Check sheet for the drawn part. Datum: minimum x, y, z corner. Units: mm. A direction names the side the tool comes from. Coordinates: 2 decimals unless noted, no trailing zeros. Write each loop counter-clockwise with the first axis right and the second up, starting at its lowest first coordinate (ties: lowest second). Pieces come first, ordered by that corner, then holes. Notation, with made-up numbers: (14, -18.75) - (57, -18.75) arc R13 cw to (57, 5.25) - close; hole circle Ø2 at (54, -4). An arc over 180 degrees is marked (long way). Use one line per item in the form item = value. Start each with the question number.
1. Cross-section at A-A on y = 4. Record the boundary of the cut face in (x, z).
2. Cross-section at C-C on z = 10.5. Record the boundary of the cut face in (x, y).
3. Scan lines: line 1 along Z through (x, y) = (56, 7.5); line 2 along Z through (x, y) = (39, 34); line 3 along X through (y, z) = (19.5, 13). Record each from-to range of solid material in increasing order.
4. Cross-section at B-B on y = 37.5. Record the boundary of the cut face in (x, z), then the cut area to 3 significant figures.
5. Tool access check on the marked faces 1, 2 and 3. Record the directions out of +Z, -Z, +X, -X, +Y, -Y that give a thin tool (end or side, any length) a straight path to the whole face; none if there is none.
6. Go/stop test with flat-tipped pins: pin 1 Ø1 at (x, z) = (43, 7.5) entering from +Y; pin 2 Ø5 at (x, y) = (8, 29.5) entering from +Z; pin 3 Ø3 at (x, z) = (63, 25.5) entering from +Y; pin 4 Ø1.5 at (y, z) = (14.5, 37.5) entering from +X. Record where each tip stops, or that it passes through.
7. Draft check along X on the marked faces 4, 5, 6 and 7. Enter one of: +X half, -X half, draft (parallel to the pull), parting line (faces both ways), or undercut.
8. Cross-section at D-D on z = 24. Record the boundary of the cut face in (x, y), then the cut area to 3 significant figures.
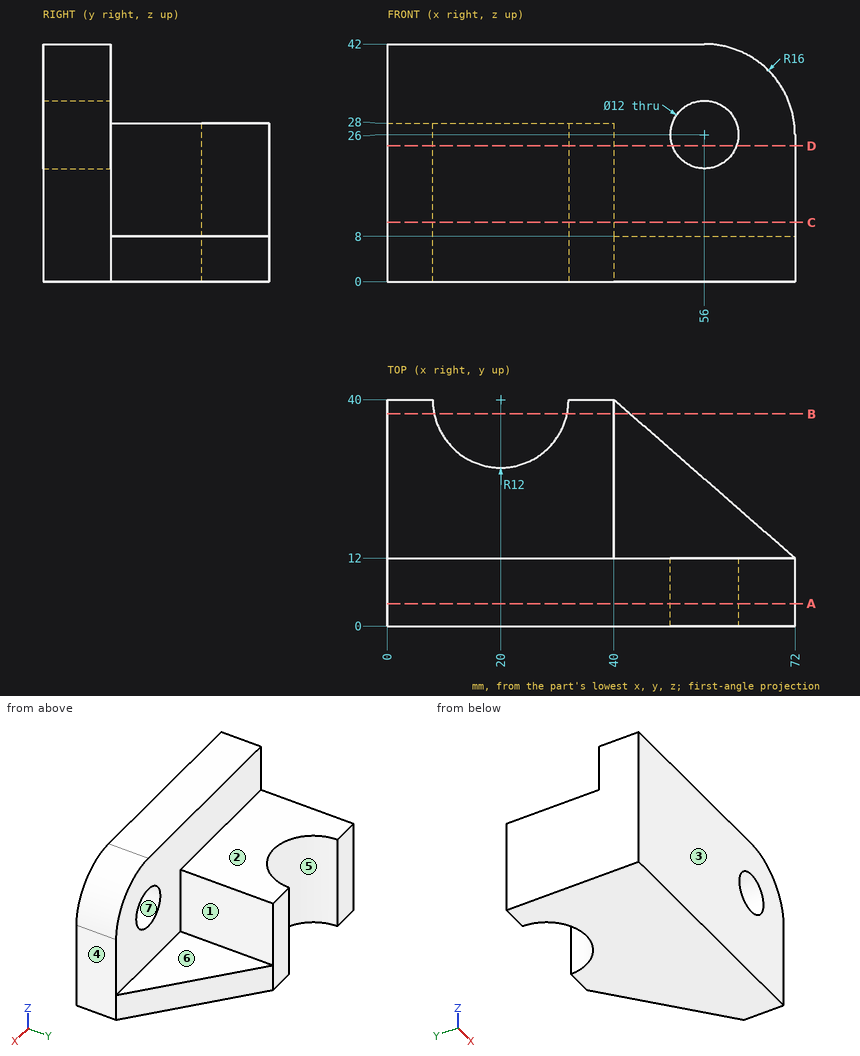
Final values:
q1.outline = (0, 0) - (72, 0) - (72, 26) arc R16 ccw to (56, 42) - (0, 42) - close; hole circle Ø12 at (56, 26)
q2.outline = (0, 0) - (72, 0) - (72, 12) - (40, 12) - (40, 40) - (32, 40) arc R12 cw to (8, 40) - (0, 40) - close
q3.line_1 = 0 to 20, 32 to 42
q3.line_2 = 0 to 28
q3.line_3 = 0 to 40
q4.outline = (0, 0) - (8.26, 0) - (8.26, 28) - (0, 28) - close; (31.74, 0) - (42.86, 0) - (42.86, 8) - (40, 8) - (40, 28) - (31.74, 28) - close
q4.area = 486 mm²
q5.face_1 = +Z, +X, +Y
q5.face_2 = +Z, +X, -X, +Y
q5.face_3 = +Z, -Z, +X, -X, -Y
q6.pin_1 = 37.81
q6.pin_2 = 28
q6.pin_3 = 12
q6.pin_4 = through
q7.face_4 = +X half
q7.face_5 = undercut
q7.face_6 = draft
q7.face_7 = undercut
q8.outline = (0, 0) - (50.34, 0) - (50.34, 12) - (40, 12) - (40, 40) - (32, 40) arc R12 cw to (8, 40) - (0, 40) - close; (61.66, 0) - (72, 0) - (72, 12) - (61.66, 12) - close
q8.area = 1,620 mm²
